Check sheet for the modelled part. Datum: model origin and axes. Units: mm. A direction names the side the tool comes from. Round coordinates to 2 decimals unless told otherwise and drop trailing zeros. Write each loop counter-clockwise with the first axis right and the second up, starting at its lowest first coordinate (ties: lowest second). Pieces come first, ordered by that corner, then holes.
from build123d import *

# Parameters (mm, degrees)
SKETCH1_W           = 150
SKETCH1_H           = 300
BOSS_EXTRUDE1_DEPTH = 110
BOSS_EXTRUDE2_DEPTH = 190
SKETCH3_W           = 101.897148024
SKETCH3_H           = 51.376713289
BOSS_EXTRUDE3_DEPTH = 100
SKETCH4_W           = 68.173568538
SKETCH4_H           = 68.173568538
BOSS_EXTRUDE4_DEPTH = 100
SKETCH5_W           = 129.298061779
SKETCH5_H           = 120.735276231
BOSS_EXTRUDE5_DEPTH = 100
SKETCH6_R           = 3
CUT_EXTRUDE1_DEPTH  = 160


with BuildPart() as part:
    # Sketch1 → Boss-Extrude1 (new body)
    with BuildSketch(Plane(origin=(0, 0, 0), x_dir=(1, 0, 0), z_dir=(0, 1, 0))):
        with Locations((75, 150)):
            Rectangle(SKETCH1_W, SKETCH1_H)
    extrude(amount=-BOSS_EXTRUDE1_DEPTH)

    # Sketch2 → Boss-Extrude2 (add)
    with BuildSketch(Plane(origin=(0, 0, 0), x_dir=(1, 0, 0), z_dir=(0, 1, 0))):
        with BuildLine():
            Line((80.063819978, 140.910835022), (138.200643085, 117.710875285))
            Line((138.200643085, 117.710875285), (138.200643085, 0))
            Line((138.200643085, 0), (186.229076195, 0))
            Line((186.229076195, 0), (189.093435683, 214.792084693))
            ThreePointArc((189.093435683, 214.792084693), (64.923783369, 280.6439946), (80.063819978, 140.910835022))
        make_face()
    extrude(amount=BOSS_EXTRUDE2_DEPTH)

    # Sketch3 → Boss-Extrude3 (add)
    with BuildSketch(Plane.ZY):
        with Locations((-118.745807749, -55.260989225)):
            Rectangle(SKETCH3_W, SKETCH3_H)
    extrude(amount=BOSS_EXTRUDE3_DEPTH)

    # Sketch4 → Boss-Extrude4 (add)
    with BuildSketch(Plane(origin=(0, -29.57263258, 0), x_dir=(1, 0, 0), z_dir=(0, 1, 0))):
        with Locations((-100, 169.694381761)):
            Rectangle(SKETCH4_W, SKETCH4_H)
    extrude(amount=BOSS_EXTRUDE4_DEPTH)

    # Sketch5 → Boss-Extrude5 (add)
    with BuildSketch(Plane(origin=(0, 70.42736742, 0), x_dir=(1, 0, 0), z_dir=(0, 1, 0))):
        with Locations((-110.357521621, 145.07637331)):
            Rectangle(SKETCH5_W, SKETCH5_H)
    extrude(amount=BOSS_EXTRUDE5_DEPTH)

    # Sketch6 → Cut-Extrude1 (cut)
    with BuildSketch(Plane.XY.offset(-84.708735194)):
        with Locations((-93.625898684, 103.612565913)):
            Circle(SKETCH6_R)
    extrude(amount=-CUT_EXTRUDE1_DEPTH, mode=Mode.SUBTRACT)


solid = part.part
1. Scan lines: line 1 along Y through (x, z) = (-95, -130); line 2 along X through (y, z) = (-6, -155.5); line 3 along Y through (x, z) = (72, -88.5). Record each from-to range of solid material in increasing order.
2. Go/stop test with flat-tipped pins: pin 1 (8 mm diameter, centred on x = -93.63, y = 103.61, fed in from -Z); pin 2 (12 mm diameter, centred on x = -26.5, z = -178.5, fed in from +Y); pin 3 (1.5 mm diameter, centred on y = 31.5, z = -82.5, fed in from +X); pin 4 (2 mm diameter, centred on x = -65, y = -17.5, fed in from -Z). Record where each tip stops, or that it passes through.
3. Set-up check for faces 1 (the flat face through (-100, -55, -119)), 2 (the flat face through (-111, 170.427, -146)), 3 (the flat face through (-111, 120, -84.709)): record each of +Z, -Z, +X, -X, +Y, -Y from which the full face is reachable in a straight line by a thin tool's end or side.
4. Release check for a two-part mould opening along Y. For faces 4 (the flat face through (-111, 70.427, -133)), 5 (the flat face through (169, 0, -144)), 6 (the flat face through (-100, 20, -135.608)), 7 (the flat face through (-45.708, 120, -144)) record: released by +Y, released by -Y, zero draft, split by the parting line, or undercut.
5. Sectioned sample at B-B, the plane z = -100. Enter the section's corners in (x, y).
6. Sectioned sample at D-D, the plane x = -81. Enter the section's corners in (y, z).
7. Sectioned sample at A-A, the plane y = 10. Enter the section's corners in (x, z).
8. Sectioned sample at C-C, the plane y = -67. Enter the section's corners in (x, z), plus the area to 3 significant figures.
Computed values:
1. line 1: y = -80.95 to -29.57, 70.43 to 100.95, 106.28 to 170.43
1. line 2: x = -134.09 to -65.91, 0 to 150
1. line 3: y = -110 to 0
2. pin 1: stops at z = -205.44
2. pin 2: passes through
2. pin 3: stops at x = 187.34
2. pin 4: stops at z = -203.78
3. face 1: +Z, -Z, -X, -Y
3. face 2: +Z, -Z, -X, +Y
3. face 3: +Z, -X, +Y
4. face 4: undercut
4. face 5: released by -Y
4. face 6: undercut
4. face 7: zero draft
5. outline: (-175.01, 70.43) - (-45.71, 70.43) - (-45.71, 170.43) - (-175.01, 170.43) - close; (-100, -80.95) - (0, -80.95) - (0, -110) - (150, -110) - (150, 0) - (187.56, 0) - (187.56, 190) - (138.2, 190) - (138.2, 0) - (0, 0) - (0, -29.57) - (-100, -29.57) - close; hole circle Ø6 at (-93.63, 103.61)
6. outline: (-80.95, -169.69) - (-29.57, -169.69) - (-29.57, -203.78) - (70.43, -203.78) - (70.43, -205.44) - (170.43, -205.44) - (170.43, -84.71) - (70.43, -84.71) - (70.43, -135.61) - (-29.57, -135.61) - (-29.57, -67.8) - (-80.95, -67.8) - close
7. outline: (-134.09, -203.78) - (-65.91, -203.78) - (-65.91, -135.61) - (-134.09, -135.61) - close; (80.06, -140.91) arc R79.55 ccw (long way) to (189.09, -214.79) - (186.23, 0) - (138.2, 0) - (138.2, -117.71) - close
8. outline: (-100, -169.69) - (0, -169.69) - (0, -300) - (150, -300) - (150, 0) - (0, 0) - (0, -67.8) - (-100, -67.8) - close
8. area: 55,200 mm2
